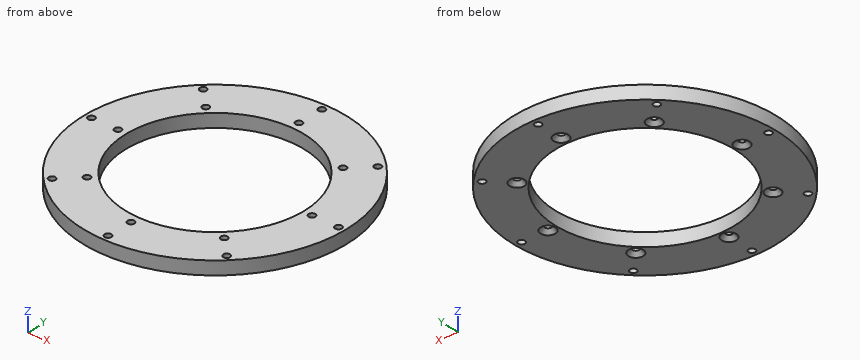
```python
from build123d import *

# Parameters (mm, degrees)
SKETCH_1_R                   = 59
SKETCH_1_R_2                 = 50.5
EXTRUDE_1_DEPTH              = 6
SKETCH_2_R                   = 1.525
CUT_EXTRUDE_1_DEPTH          = 6
EXTRUDE_START                = -6
SKETCH_6_R                   = 50.5
SKETCH_6_R_2                 = 40
EXTRUDE_2_DEPTH              = 6
SKETCH_7_R                   = 1.525
CUT_EXTRUDE_3_DEPTH          = 6
HOLE_WIZARD_M3_2_D           = 3.05
HOLE_WIZARD_M3_2_CSINK_D     = 6.6
HOLE_WIZARD_M3_2_CSINK_ANGLE = 90
PATTERN_CIRCULAR_2_COUNT     = 8


with BuildPart() as part:
    # 草图1 → 凸台-拉伸1 (new body)
    with BuildSketch(Plane.XY):
        Circle(SKETCH_1_R)
        Circle(SKETCH_1_R_2, mode=Mode.SUBTRACT)
    extrude(amount=EXTRUDE_1_DEPTH)

    # 草图2 → 切除-拉伸1 (cut)
    with BuildSketch(Plane.XY.offset(6)):
        with Locations((0, 56)):
            Circle(SKETCH_2_R)
        with Locations((39.597979746, 39.597979746)):
            Circle(SKETCH_2_R)
        with Locations((56, 0)):
            Circle(SKETCH_2_R)
        with Locations((39.597979746, -39.597979746)):
            Circle(SKETCH_2_R)
        with Locations((0, -56)):
            Circle(SKETCH_2_R)
        with Locations((-39.597979746, -39.597979746)):
            Circle(SKETCH_2_R)
        with Locations((-56, 0)):
            Circle(SKETCH_2_R)
        with Locations((-39.597979746, 39.597979746)):
            Circle(SKETCH_2_R)
    extrude(amount=-CUT_EXTRUDE_1_DEPTH, mode=Mode.SUBTRACT)

    # 草图6 → 凸台-拉伸2 (add)
    with BuildSketch(Plane.XY.offset(6).offset(EXTRUDE_START)):
        Circle(SKETCH_6_R)
        Circle(SKETCH_6_R_2, mode=Mode.SUBTRACT)
    extrude(amount=EXTRUDE_2_DEPTH)

    # 草图7 → 切除-拉伸3 (cut)
    with BuildSketch(Plane(origin=(0, 0, 0), x_dir=(-1, 0, 0), z_dir=(0, 0, -1))):
        with Locations((0, 44)):
            Circle(SKETCH_7_R)
        with Locations((31.112698372, 31.112698372)):
            Circle(SKETCH_7_R)
        with Locations((44, 0)):
            Circle(SKETCH_7_R)
        with Locations((31.112698372, -31.112698372)):
            Circle(SKETCH_7_R)
        with Locations((0, -44)):
            Circle(SKETCH_7_R)
        with Locations((-31.112698372, -31.112698372)):
            Circle(SKETCH_7_R)
        with Locations((-44, 0)):
            Circle(SKETCH_7_R)
        with Locations((-31.112698372, 31.112698372)):
            Circle(SKETCH_7_R)
    extrude(amount=-CUT_EXTRUDE_3_DEPTH, mode=Mode.SUBTRACT)

    # M3 十字槽沉头木螺钉的锥形沉头孔2 (through all)
    with Locations(Plane(origin=(0, 0, 0), x_dir=(-1, 0, 0), z_dir=(0, 0, -1))):
        with Locations((0, 44)):
            hole_wizard_m3_2 = CounterSinkHole(HOLE_WIZARD_M3_2_D / 2, HOLE_WIZARD_M3_2_CSINK_D / 2, counter_sink_angle=HOLE_WIZARD_M3_2_CSINK_ANGLE)

    # 阵列(圆周)2: M3 十字槽沉头木螺钉的锥形沉头孔2 ×8 about axis
    pattern_circular_2_axis = Axis((0, 0, 0), (0, 0, 1))
    for i in range(1, PATTERN_CIRCULAR_2_COUNT):
        add(hole_wizard_m3_2.rotate(pattern_circular_2_axis, i * 360 / PATTERN_CIRCULAR_2_COUNT), mode=Mode.SUBTRACT)


solid = part.part
```
Can you work these out from the model? Positions are in its coordinate system, mm. Give positions to 0.01 mm unless a question says otherwise; leave off trailing zeros. Loops run counter-clockwise (first coordinate to the right, second up) from the corner with the lowest first, then second, coordinate; pieces in that order, holes last. Notation, with made-up numbers: M 13.5,64 L 34.5,64 A16 cw 34.5,75 Z; hole C -6.5,-7.75 d10. An arc over 180 degrees is marked long. Answer in a Markdown table with one row per item.
1. Suppose I cut it at A-A on x = 44. Write out the boundary of the cut face in (y, z) (3 decimals), plus the area to 3 significant figures.
Taken from the geometry:
| item | result |
|---|---|
| outline | M -39.306,0 L -3.3,0 L -1.525,1.775 L -1.525,6 L -39.306,6 Z; M 1.525,1.775 L 3.3,0 L 39.306,0 L 39.306,6 L 1.525,6 Z |
| area | 450 mm² |
2. Suppose I cut it at D-D on y = 56. Write out the boundary of the cut face in (x, z) (3 decimals), plus the area to 3 significant figures.
Taken from the geometry:
| item | result |
|---|---|
| outline | M -18.574,0 L -1.525,0 L -1.525,6 L -18.574,6 Z; M 1.525,0 L 18.574,0 L 18.574,6 L 1.525,6 Z |
| area | 205 mm² |
3. Suppose I cut it at C-C on x = 0. Write out the boundary of the cut face in (y, z) (3 decimals).
Taken from the geometry:
| item | result |
|---|---|
| outline | M -59,0 L -57.525,0 L -57.525,6 L -59,6 Z; M -54.475,0 L -47.3,0 L -45.525,1.775 L -45.525,6 L -54.475,6 Z; M -42.475,1.775 L -40.7,0 L -40,0 L -40,6 L -42.475,6 Z; M 40,0 L 40.7,0 L 42.475,1.775 L 42.475,6 L 40,6 Z; M 45.525,1.775 L 47.3,0 L 54.475,0 L 54.475,6 L 45.525,6 Z; M 57.525,0 L 59,0 L 59,6 L 57.525,6 Z |
4. If I drill on line 1 along Y through (x, z) = (0, 3.75) (3 decimals); line 2 along Y through (x, z) = (32, 5); line 3 along X through (y, z) = (-23, 2.75), over which ranges is the centre line in solid material (lowest first)?
Taken from the geometry:
| item | result |
|---|---|
| line 1 | y = -59 to -57.525, -54.475 to -45.525, -42.475 to -40, 40 to 42.475, 45.525 to 54.475, 57.525 to 59 |
| line 2 | y = -49.57 to -32.35, -29.87 to -24, 24 to 29.87, 32.35 to 49.57 |
| line 3 | x = -54.33 to -32.73, 32.73 to 54.33 |
5. For pin 1 Ø1.5 at (x, z) = (-28, 4.5) entering from -Y, with a flat end and sliding along its axis, tell me the tip position at first contact or that it passes through.
Taken from the geometry:
| item | result |
|---|---|
| pin 1 | stops at y = -52.33 |
